```python
from build123d import *

# Parameters (mm, degrees)
F1_DEPTH = 1.778
F3_DEPTH = 4.572


with BuildPart() as f1:
    # F0 (on Front) → F1 (new body)
    with BuildSketch(Plane.XZ):
        with BuildLine():
            Line((-63.5, -63.5), (63.5, -63.5))
            Line((63.5, -63.5), (63.5, -9.525))
            Line((63.5, -9.525), (45.032244, -9.525))
            Line((45.032244, -9.525), (36.890166, -9.525))
            ThreePointArc((36.890166, -9.525), (24.567214, -29.121504), (3.175, -37.967478))
            Line((3.175, -37.967478), (3.175, -41.152703))
            ThreePointArc((3.175, -41.152703), (-29.185832, -29.185832), (-41.152703, 3.175))
            Line((-41.152703, 3.175), (-37.967478, 3.175))
            ThreePointArc((-37.967478, 3.175), (-29.096619, 24.596681), (-9.450293, 36.909375))
            ThreePointArc((-9.450293, 36.909375), (-7.14375, 44.400195), (0, 47.625))
            ThreePointArc((0, 47.625), (30.120695, 36.890166), (46.66278, 9.525))
            Line((46.66278, 9.525), (63.5, 9.525))
            Line((63.5, 9.525), (63.5, 63.5))
            Line((63.5, 63.5), (-63.5, 63.5))
            Line((-63.5, 63.5), (-63.5, -63.5))
        make_face()
    extrude(amount=F1_DEPTH)

    # F2 (on Front) → F3 (join)
    with BuildSketch(Plane.XZ):
        with BuildLine():
            Line((-63.5, 63.5), (-63.5, -63.5))
            Line((-63.5, -63.5), (63.5, -63.5))
            Line((63.5, -63.5), (63.5, -9.525))
            Line((63.5, -9.525), (36.890166, -9.525))
            ThreePointArc((36.890166, -9.525), (24.567214, -29.121504), (3.175, -37.967478))
            Line((3.175, -37.967478), (3.175, -41.152703))
            ThreePointArc((3.175, -41.152703), (-29.185832, -29.185832), (-41.152703, 3.175))
            Line((-41.152703, 3.175), (-37.967478, 3.175))
            ThreePointArc((-37.967478, 3.175), (-3.220369, 37.963657), (36.890166, 9.525))
            Line((36.890166, 9.525), (63.5, 9.525))
            Line((63.5, 9.525), (63.5, 63.5))
            Line((63.5, 63.5), (-63.5, 63.5))
        make_face()
    extrude(amount=-F3_DEPTH)


solid = f1.part
```
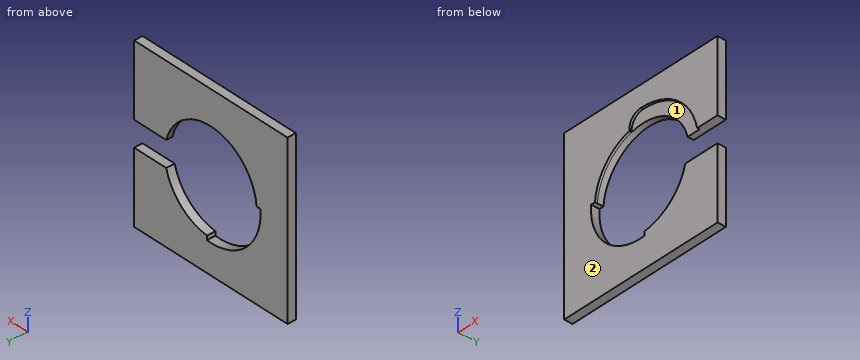
Read the model definition and answer for the solid it produces. Units are mm, in the model's axes. Face numbers are marked on the shaded views. Coordinates: 2 decimals unless noted, no trailing zeros. Order: outer loops, then holes, each group sorted by start corner. A loop starts at its lowest first (then second) coordinate and runs counter-clockwise, first axis right, second up. Notation, with made-up numbers: (44.5, 59) - (103.5, 59) arc R23 cw to (103.5, 84) - close; hole circle Ø5 at (30.25, 69). An arc over 180 degrees is marked (long way). Answer as a JSON object with one key per item and string values. Group by question number.
Item 1: Section C-C (y = 3.5) is taken. Give the vertices of the cut face in (x, z) (3 decimals).
Item 2: Section B-B (z = 31) is taken. Give the vertices of the cut face in (x, y), plus the area to 3 significant figures.
Item 3: Section D-D (x = -22) is taken. Give the vertices of the cut face in (y, z), plus the area to 3 significant figures.
Item 4: Consider probe 1 along Z at (x, y) = (44, 4.25) (3 decimals); probe 2 along X at (y, z) = (-0.5, 13); probe 3 along Z at (x, y) = (-10, 3). Determine where each line is inside the solid, lowest interval first. Write a range as from..to.
Item 5: The mould has two halves that part along Z. Classify the marked faces 1 and 2: +Z half, -Z half, draft (parallel to the pull), parting line (faces both ways), or undercut.
Item 6: Flat-ended cylindrical pins translate along their axes: P1, Ø5, axis at x = 39, z = 14.5, coming from the -Y side; P2, Ø6, axis at x = -32.5, z = -15, coming from the -Y side. Find the tip coordinate at first contact, or state that the pin passes through.
Item 7: Section A-A (x = 56) is taken. Give the vertices of the cut face in (y, z) (3 decimals), plus the area to 3 significant figures.
Results are:
{
 "1": {"outline": "(-63.5, -63.5) - (63.5, -63.5) - (63.5, -9.525) - (36.89, -9.525) arc R38.1 cw to (3.175, -37.967) - (3.175, -41.153) arc R41.275 cw to (-41.153, 3.175) - (-37.967, 3.175) arc R38.1 cw to (36.89, 9.525) - (63.5, 9.525) - (63.5, 63.5) - (-63.5, 63.5) - close"},
 "2": {"outline": "(-63.5, -1.78) - (-22.15, -1.78) - (-22.15, 4.57) - (-63.5, 4.57) - close; (22.15, 0) - (36.15, 0) - (36.15, -1.78) - (63.5, -1.78) - (63.5, 4.57) - (22.15, 4.57) - close", "area": "500 mm^2"},
 "3": {"outline": "(-1.78, -63.5) - (4.57, -63.5) - (4.57, -34.92) - (-1.78, -34.92) - close; (-1.78, 31.11) - (4.57, 31.11) - (4.57, 63.5) - (-1.78, 63.5) - close", "area": "387 mm^2"},
 "4": {"probe 1": "z = -63.5..-9.525, 9.525..63.5", "probe 2": "x = -63.5..-35.81, 45.82..63.5", "probe 3": "z = -63.5..-40.05, 36.76..63.5"},
 "5": {"face 1": "undercut", "face 2": "draft"},
 "6": {"P1": "stops at y = 0", "P2": "passes through"},
 "7": {"outline": "(-1.778, -63.5) - (4.572, -63.5) - (4.572, -9.525) - (-1.778, -9.525) - close; (-1.778, 9.525) - (4.572, 9.525) - (4.572, 63.5) - (-1.778, 63.5) - close", "area": "685 mm^2"}
}
